Can you work these out from the model? Positions are in its coordinate system, mm. Face numbers are marked on the shaded views. A direction names the side the tool comes from. Round coordinates to 2 decimals unless told otherwise and drop trailing zeros. Order: outer loops, then holes, each group sorted by start corner. A loop starts at its lowest first (then second) coordinate and runs counter-clockwise, first axis right, second up. Notation, with made-up numbers: (57, -17.75) -> (85, -17.75) arc R24 cw to (85, 6.25) -> close; hole circle Ø7 at (71.5, 33.25). An arc over 180 degrees is marked (long way). One line per item, written item: value.
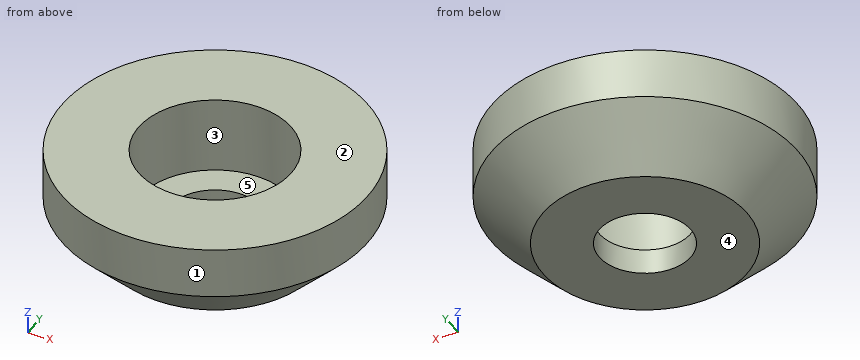
```python
from build123d import *

# Parameters (mm, degrees)
SKETCH1_R           = 3
SKETCH1_R_2         = 0.9
BOSS_EXTRUDE1_DEPTH = 2
CHAMFER1_SIZE       = 1
SKETCH2_R           = 1.5
CUT_EXTRUDE1_DEPTH  = 1.5


with BuildPart() as part:
    # Sketch1 → Boss-Extrude1 (new body)
    with BuildSketch(Plane.XY):
        Circle(SKETCH1_R)
        Circle(SKETCH1_R_2, mode=Mode.SUBTRACT)
    extrude(amount=BOSS_EXTRUDE1_DEPTH)

    # Chamfer1
    chamfer1_edges = [part.edges().sort_by_distance(p)[0] for p in [
        (-3, 0, 0),
    ]]
    chamfer(chamfer1_edges, length=CHAMFER1_SIZE)

    # Sketch2 → Cut-Extrude1 (cut)
    with BuildSketch(Plane.XY.offset(2)):
        Circle(SKETCH2_R)
    extrude(amount=-CUT_EXTRUDE1_DEPTH, mode=Mode.SUBTRACT)


solid = part.part
```
Q1. On a 3-axis mill with a long thin cutter (end or side, diameter ignored), from which of +Z, -Z, +X, -X, +Y, -Y can I reach the whole of each face in a straight line? I mean the marked faces 4 and 5. Say none if no direction works.
Answers below:
face 4: -Z, +X, -X, +Y, -Y
face 5: +Z
Q2. I want a section at D-D on z = 0.2. List the corners of the cut face in (x, y) for me, plus the area to 3 significant figures.
Answers below:
outline: circle Ø4.4 at (0, 0); hole circle Ø1.8 at (0, 0)
area: 12.7 mm^2
Q3. I want a section at C-C on z = 1.4. List the corners of the cut face in (x, y) for me.
Answers below:
outline: circle Ø6 at (0, 0); hole circle Ø3 at (0, 0)
Q4. Please list where these lines run through material, in increasing order: line 1 along Y through (x, z) = (0, 1.55); line 2 along X through (y, z) = (0.2, 0.9).
Answers below:
line 1: -3 to -1.5, 1.5 to 3
line 2: -2.89 to -1.49, 1.49 to 2.89
Q5. I want a section at A-A on y = 0. List the corners of the cut face in (x, z) for me, plus the area to 3 significant figures.
Answers below:
outline: (-3, 1) -> (-2, 0) -> (-0.9, 0) -> (-0.9, 0.5) -> (-1.5, 0.5) -> (-1.5, 2) -> (-3, 2) -> close; (0.9, 0) -> (2, 0) -> (3, 1) -> (3, 2) -> (1.5, 2) -> (1.5, 0.5) -> (0.9, 0.5) -> close
area: 5.60 mm^2
Q6. Will these pins go through, and if not, where does the flat tip stop? pin 1 Ø2 at (x, y) = (0, 0) entering from +Z; pin 2 Ø3.5 at (x, y) = (0, 0.5) entering from +Z.
Answers below:
pin 1: z = 0.5
pin 2: z = 2
Q7. We'd pull the mould along X, two halves only. Please class the marked faces 1, 2 and 3: released by +X, released by -X, zero draft, split by the parting line, or undercut.
Answers below:
face 1: split by the parting line
face 2: zero draft
face 3: undercut
